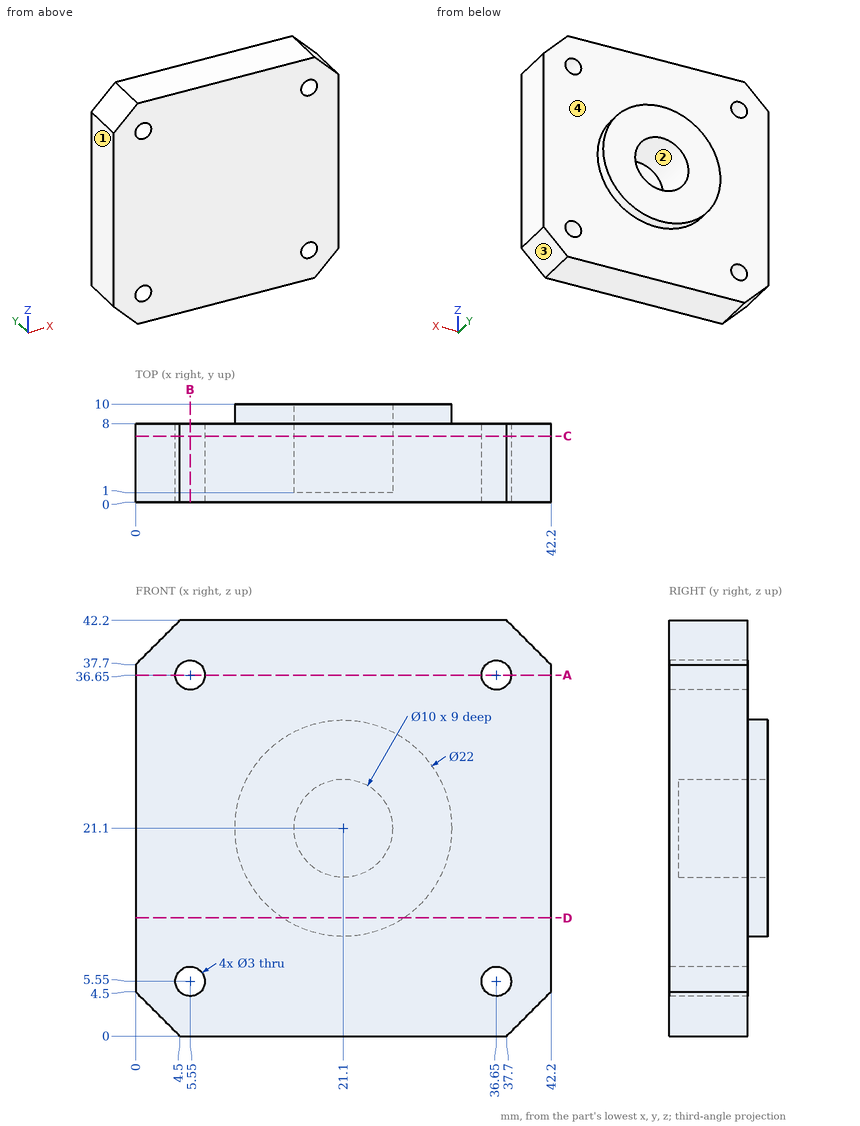
Study the drawing (mm; zero at the part's minimum x, y, z) and answer. Give positions to 0.01 mm unless a question says otherwise; leave off trailing zeros. Order: outer loops, then holes, each group sorted by start corner. A loop starts at its lowest first (then second) coordinate and runs counter-clockwise, first axis right, second up. Notation, with made-up numbers: (-25, 16.5) -> (19, 16.5) arc R23 cw to (19, 28.5) -> close; hole circle Ø1 at (34, -10.75). An arc over 180 degrees is marked (long way). Put each result on its own line as item: value.
Item 1: A cutting plane is placed at A-A on z = 36.65. Give the vertices of the cut face in (x, y), plus the area to 3 significant figures.
Established:
outline: (0, 0) -> (4.05, 0) -> (4.05, 8) -> (0, 8) -> close; (7.05, 0) -> (35.15, 0) -> (35.15, 8) -> (7.05, 8) -> close; (38.15, 0) -> (42.2, 0) -> (42.2, 8) -> (38.15, 8) -> close
area: 290 mm^2
Item 2: A cutting plane is placed at B-B on x = 5.55. Give the vertices of the cut face in (y, z).
Established:
outline: (0, 0) -> (8, 0) -> (8, 4.05) -> (0, 4.05) -> close; (0, 7.05) -> (8, 7.05) -> (8, 35.15) -> (0, 35.15) -> close; (0, 38.15) -> (8, 38.15) -> (8, 42.2) -> (0, 42.2) -> close
Item 3: Given P1, Ø6, axis at x = 27, z = 24, coming from the -Y side; P2, Ø3, axis at x = 19.5, z = 19, coming from the +Y side; P3, Ø2.5, axis at x = 36.65, z = 5.55, coming from the +Y side; P4, Ø6, axis at x = 6, z = 19, coming from the +Y side, each flat-ended and moving along its own axis, determine where each tip first touches the part or whether it passes through.
Established:
P1: stops at y = 0
P2: stops at y = 1
P3: passes through
P4: stops at y = 8
Item 4: Straight lines are drawn through the part: line 1 (Z direction, x = 36.65, y = 6); line 2 (Z direction, x = 38, y = 5.5); line 3 (Z direction, x = 21, y = 5.5). For each, find the intervals that lie inside material, in ascending order.
Established:
line 1: z = 0 to 4.05, 7.05 to 35.15, 38.15 to 42.2
line 2: z = 0.3 to 4.9, 6.2 to 36, 37.3 to 41.9
line 3: z = 0 to 16.1, 26.1 to 42.2
Item 5: A cutting plane is placed at D-D on z = 12. Give the vertices of the cut face in (x, y).
Established:
outline: (0, 0) -> (42.2, 0) -> (42.2, 8) -> (27.28, 8) -> (27.28, 10) -> (14.92, 10) -> (14.92, 8) -> (0, 8) -> close
Item 6: For a pull along X with two mould halves and no side action, classify the marked faces 1, 2, 3 and 4 as released by +X, released by -X, zero draft, split by the parting line, or undercut.
Established:
face 1: released by -X
face 2: undercut
face 3: released by +X
face 4: zero draft
Item 7: A cutting plane is placed at C-C on y = 6.75. Give the vertices of the cut face in (x, z), plus the area to 3 significant figures.
Established:
outline: (0, 4.5) -> (4.5, 0) -> (37.7, 0) -> (42.2, 4.5) -> (42.2, 37.7) -> (37.7, 42.2) -> (4.5, 42.2) -> (0, 37.7) -> close; hole circle Ø3 at (5.55, 5.55); hole circle Ø3 at (5.55, 36.65); hole circle Ø10 at (21.1, 21.1); hole circle Ø3 at (36.65, 5.55); hole circle Ø3 at (36.65, 36.65)
area: 1,630 mm^2
